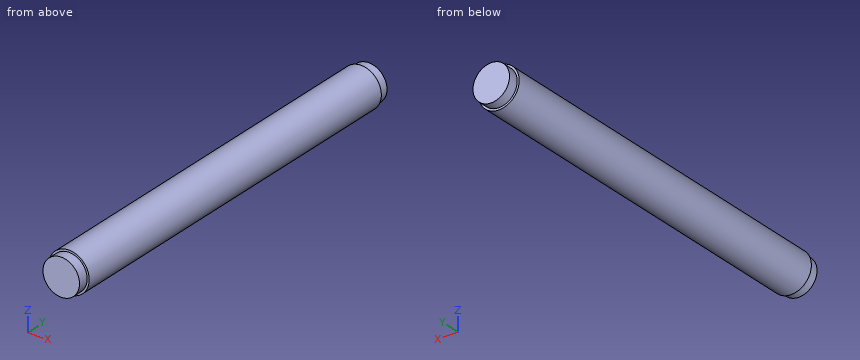
from build123d import *

# Parameters (mm, degrees)
SKETCH1_R           = 5
BOSS_EXTRUDE1_DEPTH = 100.5
SKETCH24_R          = 5
SKETCH24_R_2        = 4.5
CUT_EXTRUDE3_DEPTH  = 2.5
SKETCH25_R          = 5
SKETCH25_R_2        = 4.5
CUT_EXTRUDE4_DEPTH  = 2.5


with BuildPart() as part:
    # Sketch1 → Boss-Extrude1 (new body)
    with BuildSketch(Plane(origin=(0, 0, 0), x_dir=(1, 0, 0), z_dir=(0, 1, 0))):
        Circle(SKETCH1_R)
    extrude(amount=BOSS_EXTRUDE1_DEPTH)

    # Sketch24 → Cut-Extrude3 (cut)
    with BuildSketch(Plane(origin=(0, 0, 0), x_dir=(-1, 0, 0), z_dir=(0, -1, 0))):
        Circle(SKETCH24_R)
        Circle(SKETCH24_R_2, mode=Mode.SUBTRACT)
    extrude(amount=-CUT_EXTRUDE3_DEPTH, mode=Mode.SUBTRACT)

    # Sketch25 → Cut-Extrude4 (cut)
    with BuildSketch(Plane(origin=(0, 100.5, 0), x_dir=(1, 0, 0), z_dir=(0, 1, 0))):
        Circle(SKETCH25_R)
        Circle(SKETCH25_R_2, mode=Mode.SUBTRACT)
    extrude(amount=-CUT_EXTRUDE4_DEPTH, mode=Mode.SUBTRACT)


solid = part.part
Design review of the part built by this model. Coordinates are the model's own, in mm. Round coordinates to 2 decimals unless told otherwise and drop trailing zeros. Write each loop counter-clockwise with the first axis right and the second up, starting at its lowest first coordinate (ties: lowest second). Pieces come first, ordered by that corner, then holes. Notation, with made-up numbers: (22.25, 44.5) - (42.25, 44.5) arc R35 cw to (42.25, 78.5) - close; hole circle Ø10 at (60, 54.25). An arc over 180 degrees is marked (long way). Use a Markdown table: item, result. Add a question column.
1. We need section C-C (y = 66). State the section outline as (x, z) points.
2. We need section B-B (x = 1). State the section outline as (y, z) points.
3. Clearance check with flat-ended pins moving along their axes: pin 1 (1.5 mm diameter, centred on y = 72.5, z = -2, fed in from +X); pin 2 (1.5 mm diameter, centred on x = 3.5, y = 58.5, fed in from +Z); pin 3 (5 mm diameter, centred on x = -1.5, y = 67, fed in from -Z); pin 4 (1.5 mm diameter, centred on x = 3, y = 21, fed in from +Z). State where each tip first meets the part, or that it passes through.
4. Wall thickness on probe 1 along Z at (x, y) = (0.25, 49.5); probe 2 along Y at (x, z) = (4.5, -0.75): over which ranges is each line inside the solid? List them lowest first.
5. We need section A-A (z = 3). State the section outline as (x, y) points, then the cut area to 3 significant figures.
Output:
| question | item | result |
|---|---|---|
| 1 | outline | circle Ø10 at (0, 0) |
| 2 | outline | (0, -4.39) - (2.5, -4.39) - (2.5, -4.9) - (98, -4.9) - (98, -4.39) - (100.5, -4.39) - (100.5, 4.39) - (98, 4.39) - (98, 4.9) - (2.5, 4.9) - (2.5, 4.39) - (0, 4.39) - close |
| 3 | pin 1 | stops at x = 4.84 |
| 3 | pin 2 | stops at z = 4.18 |
| 3 | pin 3 | stops at z = -5 |
| 3 | pin 4 | stops at z = 4.47 |
| 4 | probe 1 | z = -4.99 to 4.99 |
| 4 | probe 2 | y = 2.5 to 98 |
| 5 | outline | (-4, 2.5) - (-3.35, 2.5) - (-3.35, 0) - (3.35, 0) - (3.35, 2.5) - (4, 2.5) - (4, 98) - (3.35, 98) - (3.35, 100.5) - (-3.35, 100.5) - (-3.35, 98) - (-4, 98) - close |
| 5 | area | 798 mm2 |
